from build123d import *

# Parameters (mm, degrees)
F1_DEPTH = 25.4
F2_R     = 4.7625
F3_DEPTH = 12.701
F4_R     = 4.7625
F5_DEPTH = 12.701
F6_R     = 4
F7_DEPTH = 25.401
F8_R     = 3.175
F9_DEPTH = 3.175


with BuildPart() as f1:
    # F0 (on Front) → F1 (new body)
    with BuildSketch(Plane.XZ):
        Polygon((-31.75, 12.7), (-31.75, 0), (31.75, 0), (31.75, 12.7), (12.7, 12.7), (12.7, 38.1), (-12.7, 38.1), (-12.7, 12.7), align=None)
    extrude(amount=F1_DEPTH)

    # F2 (on face) → F3 (cut, through all)
    with BuildSketch(Plane.XY.offset(12.7)):
        with Locations((-22.225, -12.7)):
            Circle(F2_R)
    extrude(amount=-F3_DEPTH, mode=Mode.SUBTRACT)

    # F4 (on face) → F5 (cut, through all)
    with BuildSketch(Plane.XY.offset(12.7)):
        with Locations((22.225, -12.7)):
            Circle(F4_R)
    extrude(amount=-F5_DEPTH, mode=Mode.SUBTRACT)

    # F6 (on face) → F7 (cut, through all)
    with BuildSketch(Plane.XZ.offset(25.4)):
        with Locations((0, 25.4)):
            Circle(F6_R)
    extrude(amount=-F7_DEPTH, mode=Mode.SUBTRACT)

    # F8 (on face) → F9 (cut)
    with BuildSketch(Plane(origin=(0, 0, 0), x_dir=(1, 0, 0), z_dir=(0, 0, -1))):
        with Locations((0, 12.7)):
            Circle(F8_R)
    extrude(amount=-F9_DEPTH, mode=Mode.SUBTRACT)


solid = f1.part
Check sheet for the modelled part. Datum: model origin and axes. Units: mm. A direction names the side the tool comes from. Coordinates: 2 decimals unless noted, no trailing zeros. Write each loop counter-clockwise with the first axis right and the second up, starting at its lowest first coordinate (ties: lowest second). Pieces come first, ordered by that corner, then holes.
Item 1: Cross-section at A-A on z = 25.4. Record the boundary of the cut face in (x, y), then the cut area to 3 significant figures.
Numbers:
outline: (-12.7, -25.4) - (-4, -25.4) - (-4, 0) - (-12.7, 0) - close; (4, -25.4) - (12.7, -25.4) - (12.7, 0) - (4, 0) - close
area: 442 mm2
Item 2: Cross-section at C-C on y = -3.25. Record the boundary of the cut face in (x, z), then the cut area to 3 significant figures.
Numbers:
outline: (-31.75, 0) - (31.75, 0) - (31.75, 12.7) - (12.7, 12.7) - (12.7, 38.1) - (-12.7, 38.1) - (-12.7, 12.7) - (-31.75, 12.7) - close; hole circle Ø8 at (0, 25.4)
area: 1,400 mm2
Item 3: Cross-section at D-D on z = 9.5. Count the separate pieces of the cut face and the enclosed holes in it, then the cut area to 3 significant figures.
Numbers:
separate pieces: 1
enclosed holes: 2
area: 1,470 mm2
Item 4: Access from +Z, -Z, +X, -X, +Y, -Y to the whole of each face (thin tool, end or side, straight path). Record for faces 5 (the face through (0, -13, 3.175)), 6 (the face through (-12.7, -13, 26)), 7 (the face through (12.7, -13, 25)).
Numbers:
face 5: -Z
face 6: +Z, -X, +Y, -Y
face 7: +Z, +X, +Y, -Y
Item 5: Depth check by flat-ended pin: pin 1 Ø3 at (x, y) = (0.5, -12.5) entering from -Z (3 decimals); pin 2 Ø5.5 at (x, y) = (25.5, -8) entering from +Z; pin 3 Ø8 at (y, z) = (-7.5, 33.5) entering from -X. Enter the tip coordinate at first touch or a pass-through.
Numbers:
pin 1: stops at z = 3.175
pin 2: stops at z = 12.7
pin 3: stops at x = -12.7
Item 6: Scan lines: probe 1 along Y at (x, z) = (0, 1.65) (3 decimals); probe 2 along Z at (x, y) = (23, -19.5); probe 3 along X at (y, z) = (-15.75, 17). Record each from-to range of solid material in increasing order.
Numbers:
probe 1: y = -25.4 to -15.875, -9.525 to 0
probe 2: z = 0 to 12.7
probe 3: x = -12.7 to 12.7
Item 7: Cross-section at B-B on x = 0. Record the boundary of the cut face in (y, z) (3 decimals).
Numbers:
outline: (-25.4, 0) - (-15.875, 0) - (-15.875, 3.175) - (-9.525, 3.175) - (-9.525, 0) - (0, 0) - (0, 21.4) - (-25.4, 21.4) - close; (-25.4, 29.4) - (0, 29.4) - (0, 38.1) - (-25.4, 38.1) - close
Item 8: Mould release check, pull along Y, two halves, no side actions. Record for faces 1 (the face through (1.5, -9.9, 1.6)), 2 (the face through (0, -13, 38.1)), 3 (the face through (0, 0, 15)), 4 (the face through (0, -25.4, 15)): released by +Y, released by -Y, zero draft, split by the parting line, or undercut.
Numbers:
face 1: undercut
face 2: zero draft
face 3: released by +Y
face 4: released by -Y
